from build123d import *

# Parameters (mm, degrees)
SKETCH_1_R          = 8
EXTRUDE_1_DEPTH     = 43
SKETCH_2_W          = 4
SKETCH_2_H          = 20
CUT_EXTRUDE_1_DEPTH = 21.5
FILLET_1_R          = 3
FILLET_2_R          = 4
SKETCH_3_R          = 4
CUT_EXTRUDE_2_DEPTH = 21.5
SKETCH_4_R          = 4
CUT_EXTRUDE_3_DEPTH = 20


with BuildPart() as part:
    # 草图1 → 凸台-拉伸1 (new body)
    with BuildSketch(Plane(origin=(0, 0, 0), x_dir=(1, 0, 0), z_dir=(0, 1, 0))):
        with Locations(Location((0, 0, 0), (0, 0, 270))):
            Circle(SKETCH_1_R)
    extrude(amount=EXTRUDE_1_DEPTH)

    # 草图2 → 切除-拉伸1 (cut, symmetric)
    with BuildSketch(Plane(origin=(0, 0, 0), x_dir=(0, 0, -1), z_dir=(1, 0, 0))):
        with Locations((-6, 33)):
            Rectangle(SKETCH_2_W, SKETCH_2_H)
        with Locations((6, 33)):
            Rectangle(SKETCH_2_W, SKETCH_2_H)
    extrude(amount=CUT_EXTRUDE_1_DEPTH, both=True, mode=Mode.SUBTRACT)

    # 圆角1
    fillet_1_edges = [part.edges().sort_by_distance(p)[0] for p in [
        (-4, 23, 6.92820323),
        (0, 23, -8),
    ]]
    fillet(fillet_1_edges, radius=FILLET_1_R)

    # 圆角2
    fillet_2_edges = [part.edges().sort_by_distance(p)[0] for p in [
        (8, 43, 0),
        (-8, 43, 0),
    ]]
    fillet(fillet_2_edges, radius=FILLET_2_R - 0.0001)  # a hair under: the kernel refuses the full size

    # 草图3 → 切除-拉伸2 (cut, symmetric)
    with BuildSketch(Plane.XY.offset(4)):
        with Locations(Location((0, 35, 0), (0, 0, 90))):
            Circle(SKETCH_3_R)
    extrude(amount=CUT_EXTRUDE_2_DEPTH, both=True, mode=Mode.SUBTRACT)

    # 草图4 → 切除-拉伸3 (cut)
    with BuildSketch(Plane.XZ):
        with Locations(Location((0, 0, 0), (0, 0, 270))):
            Circle(SKETCH_4_R)
    extrude(amount=-CUT_EXTRUDE_3_DEPTH, mode=Mode.SUBTRACT)


solid = part.part
Source: CAD feature listing. Evaluate the final solid. Frame: model axes, mm. A direction names the side the tool comes from. Round coordinates to 2 decimals unless told otherwise and drop trailing zeros. Loops run counter-clockwise (first coordinate to the right, second up) from the corner with the lowest first, then second, coordinate; pieces in that order, holes last.
Q1. Ray query, line 1 (X direction, y = 6, z = 0); line 2 (Y direction, x = 3.5, z = 1); line 3 (Y direction, x = -0.75, z = -1.5). Return the intervals inside material, ascending.
Q2. Section A-A, the plane y = 35. Return loops of the section in (x, z).
Q3. First-contact query: P1, Ø4, axis at x = 2.5, y = 28.5, coming from the +Z side; P2, Ø3, axis at y = 30.5, z = 4.5, coming from the +X side; P3, Ø5, axis at x = 0, z = 0, coming from the -Y side. Flat tips, straight axial feed; report the tip coordinate or a pass-through.
Q4. Section C-C, the plane y = 14.5. Return loops of the section in (x, z).
Q5. Section D-D, the plane y = 28. Return loops of the section in (x, z), plus the area to 3 significant figures.
Q6. Mould query, pull axis X, two halves, no side actions, for faces 1 (the face through (-7.1, 14.89, 3.69)), 2 (the face through (0, 20, 0)), 3 (the face through (2, 31, -4)). Classes: pulls with the +X half, pulls with the -X half, needs draft (parallel to the pull), parting line crosses it, or undercut.
Q7. Access query for faces 4 (the face through (0, 23, -4.4)), 5 (the face through (0, 23, 4.4)), 6 (the face through (2.4, 31.8, 0.1)), 7 (the face through (-3.905, 9.86, 0.867)). Directions: +Z, -Z, +X, -X, +Y, -Y. A direction counts if a zero-diameter tool reaches every point of the face in a straight line with its end or side. Return the directions, or none.
Q8. Section B-B, the plane z = 0. Return loops of the section in (x, y).
Solutions:
1. line 1: x = -8 to -4, 4 to 8
1. line 2: y = 20 to 33.06, 36.94 to 43
1. line 3: y = 20 to 31.07, 38.93 to 43
2. outline: (-6.93, -4) - (-4, -4) - (-4, 4) - (-6.93, 4) arc R8 ccw to start; (4, -4) - (6.93, -4) arc R8 ccw to (6.93, 4) - (4, 4) - close
3. P1: stops at z = 4
3. P2: stops at x = 7.42
3. P3: stops at y = 20
4. outline: circle Ø16 at (0, 0); hole circle Ø8 at (0, 0)
5. outline: (-6.93, -4) - (6.93, -4) arc R8 ccw to (6.93, 4) - (-6.93, 4) arc R8 ccw to start
5. area: 122 mm2
6. face 1: parting line crosses it
6. face 2: undercut
6. face 3: needs draft
7. face 4: -Z, +X, -X, +Y
7. face 5: +Z, +X, -X, +Y
7. face 6: +Z, -Z
7. face 7: -Y
8. outline: (-8, 0) - (-4, 0) - (-4, 20) - (4, 20) - (4, 0) - (8, 0) - (8, 39) arc R4 ccw to (4, 43) - (-4, 43) arc R4 ccw to (-8, 39) - close; hole circle Ø8 at (0, 35)
